Geometry check sheet. Reference: the model listing, model coordinates, mm. A direction names the side the tool comes from. Give positions to 0.01 mm unless a question says otherwise; leave off trailing zeros. Loops run counter-clockwise (first coordinate to the right, second up) from the corner with the lowest first, then second, coordinate; pieces in that order, holes last. Notation, with made-up numbers: (0, 20) -> (6, 20) arc R10 ccw to (6, 24) -> close; hole circle Ø2 at (-7, 30.5). An arc over 180 degrees is marked (long way). Write each question's results on one line, items separated by ' | '. Start each with the question number.
1) Sectioned sample at D-D on x = 2. Record the cut outline in (y, z), then the cut area to 3 significant figures.
2) Depth check by flat-ended pin: pin 1 (8 mm diameter, centred on y = 27.5, z = 21.5, fed in from -X); pin 2 (4 mm diameter, centred on x = 8.5, z = -5.5, fed in from +Y); pin 3 (3 mm diameter, centred on x = 7, y = 23, fed in from -Z). Enter the tip coordinate at first touch or a pass-through.
3) Scan lines: line 1 (Z direction, x = 11.5, y = 0) (3 decimals); line 2 (Y direction, x = 5.25, z = 4); line 3 (Y direction, x = 8, z = 6). Record each from-to range of solid material in increasing order. Write a range as from..to.
4) Set-up check for faces 1 (the face through (8.05, 6.8, -8.87)), 2 (the face through (14.351, 19, 1)), 3 (the face through (3.251, 19, -1)): record each of +Z, -Z, +X, -X, +Y, -Y from which the full face is reachable in a straight line by a thin tool's end or side.
5) Sectioned sample at C-C on z = -29. Record the cut outline in (x, y).
6) Sectioned sample at A-A on z = 0. Count the separate pieces of the cut face and the enclosed holes in it, then the cut area to 3 significant figures.
```python
from build123d import *

# Parameters (mm, degrees)
F2_R     = 7.9375
F3_DEPTH = 14.352


with BuildPart() as f1:
    # F0 (on Front) → F1 (revolve)
    with BuildSketch(Plane.XZ):
        Polygon((0, 15.0876), (0, 11.176), (15.875, 11.176), (15.875, 17.4625), (14.351, 17.4625), (14.351, 44.45), (3.2512, 44.45), (3.2512, 15.0876), align=None)
    revolve(axis=Axis((0.385378, 0, 0), (1, 0, 0)))

    # F2 (on face) → F3 (cut, through all)
    with BuildSketch(Plane.YZ.offset(14.351)):
        with Locations((0, 30.1625)):
            Circle(F2_R)
        with Locations((0, -30.1625)):
            Circle(F2_R)
        with Locations((-30.1625, 0)):
            Circle(F2_R)
        with Locations((30.1625, 0)):
            Circle(F2_R)
    extrude(amount=-F3_DEPTH, mode=Mode.SUBTRACT)


solid = f1.part
```
Result:
1) outline: circle Ø30.18 at (0, 0); hole circle Ø22.35 at (0, 0) | area: 323 mm^2
2) pin 1: x = 3.25 | pin 2: y = 44.31 | pin 3: z = -38.9
3) line 1: -44.45..-38.1, -22.225..-11.176, 11.176..22.225, 38.1..44.45 | line 2: -44.27..-37.02, -23.31..-10.44, 10.44..23.31, 37.02..44.27 | line 3: -44.04..-35.36, -24.97..-9.43, 9.43..24.97, 35.36..44.04
4) face 1: +X, -X | face 2: +X | face 3: -X
5) outline: (3.25, -33.69) -> (14.35, -33.69) -> (14.35, -7.85) -> (3.25, -7.85) -> close; (3.25, 7.85) -> (14.35, 7.85) -> (14.35, 33.69) -> (3.25, 33.69) -> close
6) separate pieces: 4 | enclosed holes: 0 | area: 431 mm^2
